Autodesk Inventor part; units mm, degrees
ref_plane "YZ Plane" through (0, 0, 0) normal (1, 0, 0) x (0, 1, 0)
ref_plane "XZ Plane" through (0, 0, 0) normal (0, 1, 0) x (-1, 0, 0)
ref_plane "XY Plane" through (0, 0, 0) normal (0, 0, 1) x (1, 0, 0)
sketch "Sketch1" plane through (0, 0, 0) normal (0, 0, 1) x (1, 0, 0)
  circle A0 centre (0, 0) radius 10.75
  circle A1 centre (0, 0) radius 5.5
  line L0 (0, 0) -> (21.75, 0) construction
  line L1 (0, 0) -> (-21.75, 0) construction
  circle A2 centre (0, 0) radius 4
  circle A3 centre (21.75, 0) radius 2.75
  circle A4 centre (-21.75, 0) radius 2.75
  arc A5 (-23.0776, 5.3374) -> (-23.0776, -5.3374) centre (-21.75, 0) ccw
  line L2 (-21.75, 0) -> (-21.75, -5.5) construction
  line L3 (-21.75, 0) -> (-21.75, 5.5) construction
  arc A6 (23.0776, -5.3374) -> (23.0776, 5.3374) centre (21.75, 0) ccw
  line L4 (21.75, 0) -> (21.75, -5.5) construction
  line L5 (21.75, 0) -> (21.75, 5.5) construction
  line L6 (-23.0776, 5.3374) -> (-2.5948, 10.4321)
  line L7 (2.5948, 10.4321) -> (23.0776, 5.3374)
  line L8 (23.0776, -5.3374) -> (2.5948, -10.4321)
  line L9 (-23.0776, -5.3374) -> (-2.5948, -10.4321)
  dimension "d0" = 21.5
  dimension "d1" = 11
  dimension "d2" = 21.75
  dimension "d3" = 21.75
  dimension "d4" = 8
  dimension "d5" = 5.5
  dimension "d6" = 5.5
  dimension "d7" = 5.5
  dimension "d8" = 180
  dimension "d9" = 5.5
  dimension "d10" = 180
extrude "Extrusion1" add sketch "Sketch1" along normal blind 5.5 contours A0 | A0 L7 A6 L8 | A0 L9 A5 L6 | A1
extrude "Extrusion2" add sketch "Sketch1" along normal blind 13.5 contours A0 | A1
extrude "Extrusion3" add sketch "Sketch1" along normal blind 16.5 contours A0
sketch "Sketch2" plane through (0, 0, 5.5) normal (0, 0, 1) x (1, 0, 0)
  line L0 (-17.5, 1) -> (-10.5, 1)
  line L1 (-10.5, 1) -> (-10.5, -1)
  line L2 (-10.5, -1) -> (-17.5, -1)
  line L3 (-17.5, -1) -> (-17.5, 1)
  line L4 (-17.5, 1) -> (-10.5, -1) construction
  line L5 (-10.5, 1) -> (-17.5, -1) construction
  line L6 (10.5, 1) -> (17.5, 1)
  line L7 (17.5, 1) -> (17.5, -1)
  line L8 (17.5, -1) -> (10.5, -1)
  line L9 (10.5, -1) -> (10.5, 1)
  line L10 (10.5, 1) -> (17.5, -1) construction
  line L11 (17.5, 1) -> (10.5, -1) construction
  circle A0 centre (0, 0) radius 10.75
  point P0 (-14, 0)
  point P1 (14, 0)
  dimension "d20" = 7
  dimension "d21" = 7
  dimension "d22" = 2
  dimension "d23" = 0
  dimension "d24" = 2
  dimension "d25" = 10.5
  dimension "d26" = 10.5
extrude "Extrusion4" cut sketch "Sketch2" along normal blind 9.5 contours L0 A0 L2 L3 | L0 L1 L2 A0 | A0 L8 L9 L6 | L6 L7 L8 A0
sketch "Sketch3" plane through (10.5, -1, 5.5) normal (1, 0, 0) x (0, 0, -1)
  line L0 (-9.5, 2) -> (0, 2)
  line L1 (0, 0) -> (-9.5, 0)
  line L2 (-9.5, 2) -> (0, 2)
  line L3 (0, 2) -> (0, 0)
  line L4 (0, 0) -> (-9.5, 0)
  line L5 (-9.5, 0) -> (-9.5, 2)
  point P0 (5.5, 1)
  dimension "d29" = 9.5
  dimension "d30" = 2
sketch "Sketch4" plane through (-10.5, -1, 5.5) normal (-1, 0, 0) x (0, 0, 1)
  line L0 (9.5, 0) -> (0, 0)
  line L1 (0, 0) -> (0, 2)
  line L2 (0, 2) -> (9.5, 2)
  line L3 (9.5, 2) -> (9.5, 0)
  point P0 (-5.5, 1)
extrude "Extrusion5" add sketch "Sketch2" along normal blind 1.5 contours L0 A0 L2 L3 | L0 L1 L2 A0 | A0 L8 L9 L6 | L6 L7 L8 A0
extrude "Extrusion6" add sketch "Sketch4" along normal blind 1.5
extrude "Extrusion7" add sketch "Sketch3" along normal blind 1.5
sketch "Sketch5" plane through (10.7034, -1, 5.5) normal (0, -1, 0) x (1, 0, 0)
  line L0 (1.2966, 1.5) -> (1.2966, 9.5)
  line L1 (6.7966, 1.5) -> (1.2966, 1.5)
  line L2 (1.2966, 9.5) -> (6.7966, 1.5)
  line L3 (6.7966, 1.5) -> (1.2966, 1.5)
  line L4 (1.2966, 1.5) -> (1.2966, 9.5)
  line L5 (-22.7034, 9.5) -> (-22.7034, 1.5)
  line L6 (-28.2034, 0) -> (-28.2034, 1.5)
  line L7 (-22.7034, 9.5) -> (-28.2034, 1.5)
  line L8 (-22.7034, 1.5) -> (-28.2034, 1.5)
  line L9 (-28.2034, 1.5) -> (-22.7034, 1.5)
  line L10 (-22.7034, 1.5) -> (-22.7034, 9.5)
  point P0 (-10.7034, -5.5)
extrude "Extrusion8" add sketch "Sketch5" against normal blind 2
equation "\"d3\" = d2"
equation "\"d6\" = d5"
equation "\"d7\" = d5"
equation "\"d9\" = d5"
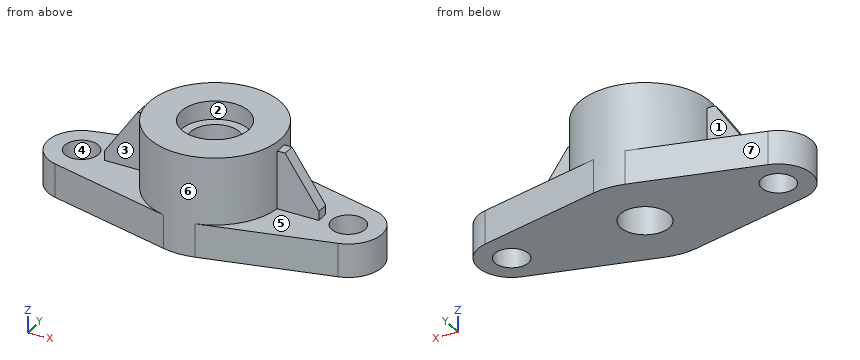
Check sheet for the modelled part. Datum: model origin and axes. Units: mm. Face numbers are marked on the shaded views. A direction names the side the tool comes from. Round coordinates to 2 decimals unless told otherwise and drop trailing zeros. Write each loop counter-clockwise with the first axis right and the second up, starting at its lowest first coordinate (ties: lowest second). Pieces come first, ordered by that corner, then holes. Notation, with made-up numbers: (83.25, -35.5) - (91.25, -35.5) arc R28 cw to (91.25, -16.5) - close; hole circle Ø9 at (39.25, 24.25). An arc over 180 degrees is marked (long way). Return JSON: item names as keys, results as strings.
Q1. Cross-section at D-D (z = 12). Record the boundary of the cut face in (x, y).
Returned:
{"outline": "(-14.06, -1) - (-10.7, -1) arc R10.75 ccw to (10.7, -1) - (14.06, -1) - (14.06, 1) - (10.7, 1) arc R10.75 ccw to (-10.7, 1) - (-14.06, 1) - close; hole circle Ø8 at (0, 0)"}
Q2. Depth check by flat-ended pin: P1, Ø3, axis at x = 8, z = 11, coming from the +Y side; P2, Ø5.5, axis at x = 13.5, z = 12.5, coming from the -Y side; P3, Ø8, axis at y = 6, z = 2, coming from the +X side. Enter the tip coordinate at first touch or a pass-through.
Returned:
{"P1": "stops at y = 8.56", "P2": "stops at y = -1", "P3": "stops at x = 26.87"}
Q3. Draft check along Y on the marked faces 4, 5, 6 and 7. Enter one of: released by +Y, released by -Y, zero draft, split by the parting line, or undercut.
Returned:
{"face 4": "undercut", "face 5": "zero draft", "face 6": "split by the parting line", "face 7": "released by +Y"}
Q4. Access from +Z, -Z, +X, -X, +Y, -Y to the whole of each face (thin tool, end or side, straight path). Record for the marked faces 1, 2 and 3.
Returned:
{"face 1": "+Z, -X, +Y", "face 2": "+Z", "face 3": "+Z, -X, -Y"}
Q5. Cross-section at A-A (y = 0). Give the number of separate pieces and of enclosed holes in the cut face, then the cut area to 3 significant figures.
Returned:
{"separate pieces": "4", "enclosed holes": "0", "area": "419 mm²"}
Q6. Cross-section at B-B (x = 0). Record the boundary of the cut face in (y, z), then the cut area to 3 significant figures.
Returned:
{"outline": "(-10.75, 0) - (-4, 0) - (-4, 13.5) - (-5.5, 13.5) - (-5.5, 16.5) - (-10.75, 16.5) - close; (4, 0) - (10.75, 0) - (10.75, 16.5) - (5.5, 16.5) - (5.5, 13.5) - (4, 13.5) - close", "area": "214 mm²"}
Q7. Scan lines: L1, parallel to Y at x = 0, z = 7.25; L2, parallel to Z at x = -16.5, y = 5.25; L3, parallel to Y at x = 0, z = 15.6. Record each from-to range of solid material in increasing order. Write a range as from..to.
Returned:
{"L1": "y = -10.75..-4, 4..10.75", "L2": "z = 0..5.5", "L3": "y = -10.75..-5.5, 5.5..10.75"}
Q8. Cross-section at C-C (z = 1.5). Record the boundary of the cut face in (x, y).
Returned:
{"outline": "(-23.08, -5.34) - (-2.59, -10.43) arc R10.75 ccw to (2.59, -10.43) - (23.08, -5.34) arc R5.5 ccw to (23.08, 5.34) - (2.59, 10.43) arc R10.75 ccw to (-2.59, 10.43) - (-23.08, 5.34) arc R5.5 ccw to start; hole circle Ø5.5 at (-21.75, 0); hole circle Ø8 at (0, 0); hole circle Ø5.5 at (21.75, 0)"}
